The model under review builds one solid part; all positions refer to its coordinate system, in mm. A direction names the side the tool comes from. Round coordinates to 2 decimals unless told otherwise and drop trailing zeros. Use one line per item in the form item = value.
from build123d import *

# Parameters (mm, degrees)
REVOLVE_ONTO_SKETCH002_ROLL_ANGLE = 90.0000000001
ARRAY_COUNT                       = 2
SKETCH001_R                       = 2
POCKET_DEPTH                      = 9.6459047106
POCKET001_DEPTH                   = 2.6
POCKET002_DEPTH                   = 5
SKETCH005_R                       = 1.7
POCKET003_DEPTH                   = 3
SKETCH006_R                       = 1.7
POCKET004_DEPTH                   = 7.3269450049


with BuildPart() as array:
    # Sketch002 as drawn → Revolve (revolve)
    with BuildSketch(Plane.XY):
        Polygon((7.25, 10), (7.25, 4), (8.5, 4), (8.5, -1), (10, -1), (10, 10), align=None)
    revolve(axis=Axis((10, -1, 0), (0, 1, 0)))


with BuildPart() as array_1:
    # Revolve onto Sketch002 roll: moved
    add(array.part.rotate(Axis((0, 0, 0), (1, 0, 0)), REVOLVE_ONTO_SKETCH002_ROLL_ANGLE))


with BuildPart() as array_2:
    # Revolve onto Sketch002 placement: moved
    add(array_1.part)

    # Array: Array ×2 about axis
    array_axis = Axis((0, 0, 0), (0, 0, 1))


with BuildPart() as array_3:
    add(array_2.part)
    for i in range(1, ARRAY_COUNT):
        add(array_2.part.rotate(array_axis, i * 360 / ARRAY_COUNT))


with BuildPart() as pocket004:
    # Sketch → Revolution (revolve)
    with BuildSketch(Plane.XZ):
        Polygon((0, 0), (15, 0), (15, 9.6449047106), (0, 7), align=None)
    revolve(axis=Axis((0, 0, 0), (0, 0, 1)))

    # Sketch001 → Pocket (cut, through all)
    with BuildSketch(Plane(origin=(0, 0, 0), x_dir=(1, 0, 0), z_dir=(0, 0, -1))):
        Circle(SKETCH001_R)
    extrude(amount=-POCKET_DEPTH, mode=Mode.SUBTRACT)

    # Cut: cut Array
    add(array_3.part, mode=Mode.SUBTRACT)

    # Sketch003 → Pocket001 (cut)
    with BuildSketch(Plane(origin=(0, 0, 0), x_dir=(1, 0, 0), z_dir=(0, 0, -1))):
        Polygon((-12.4316043172, 8.7547471036), (-8.7815991184, 12.458456332), (12.5853843422, -8.5987044497), (8.9353791434, -12.3024136782), align=None)
    extrude(amount=-POCKET001_DEPTH, mode=Mode.SUBTRACT)

    # Sketch004 → Pocket002 (cut)
    with BuildSketch(Plane(origin=(0, 0, 0), x_dir=(1, 0, 0), z_dir=(0, 0, -1))):
        Polygon((-6.9172433584, -3.9560102728), (-3.8989698287, -0.8933276416), (-0.8362871974, -3.9116011713), (-3.8545607272, -6.9742838025), align=None)
    extrude(amount=-POCKET002_DEPTH, mode=Mode.SUBTRACT)

    # Sketch005 → Pocket003 (cut)
    with BuildSketch(Plane(origin=(-2.367628513, 2.4024644064, 0), x_dir=(-0.7122517747, -0.7019240767, 0), z_dir=(-0.7019240767, 0.7122517747, 0))):
        with Locations((0, 2.8)):
            Circle(SKETCH005_R)
    extrude(amount=-POCKET003_DEPTH, mode=Mode.SUBTRACT)

    # Sketch006 → Pocket004 (cut)
    with BuildSketch(Plane(origin=(-5.3859020428, 5.4651470377, 0), x_dir=(0.7122517747, 0.7019240767, 0), z_dir=(0.7019240767, -0.7122517747, 0))):
        with Locations((0, 2.8)):
            Circle(SKETCH006_R)
    extrude(amount=-POCKET004_DEPTH, mode=Mode.SUBTRACT)


solid = pocket004.part
(1) Insertion check: P1, Ø2, axis at y = -9.5, z = 3.5, coming from the +X side; P2, Ø5, axis at x = 7.5, z = 8.5, coming from the +Y side; P3, Ø5, axis at x = -10, y = 0, coming from the +Z side; P4, Ø2.5, axis at x = 0, y = 0, coming from the -Z side. Each pin has a flat end and moves straight along its axis. Give the tip position at first contact, or say it passes through.
Geometry results:
P1 = 12.36
P2 = 14.14
P3 = 4
P4 = through
(2) To check wall thickness, follow L1, parallel to Y at x = 0, z = 4.2; L2, parallel to X at y = -1, z = 8.5; L3, parallel to Y at x = -7, z = 1.75. State the ranges of each line that lie inside material, in increasing order.
Geometry results:
L1 = -15 to -2, 2 to 15
L2 = -14.97 to -12.56, 12.56 to 14.97
L3 = -13.27 to -10.7, -3.4 to 5.2, 9.01 to 13.27
(3) The part is to be moulded in two halves that separate along Z. For faces 1 (the flat face through (-8.8, -1.2, 4)), 2 (the cylindrical face through (-1.588, 1.927, 4.486)), 3 (the flat face through (-5.36, 5.49, 0.8)), say which applies: +Z half, -Z half, draft (parallel to the pull), parting line (faces both ways), or undercut.
Geometry results:
face_1 = +Z half
face_2 = undercut
face_3 = draft
(4) Machinability: for faces 4 (the flat face through (8.8, 1.2, 4)), 5 (the cylindrical face through (1.075, -1.686, 4.943)), 6 (the flat face through (-5.429, 2.446, 2.465)), which of the approach directions +Z, -Z, +X, -X, +Y, -Y give a long, thin tool a straight path to every point of the face, cutting with its end or side? Answer none if there is none.
Geometry results:
face_4 = +Z
face_5 = +Z, -Z
face_6 = -Z
(5) Add section A-A on y = 0. Count the separate pieces of the cut face and the enclosed holes in it, then the cut area to 3 significant figures.
Geometry results:
separate_pieces = 4
enclosed_holes = 0
area = 135 mm2
